The model under review builds one solid part; all positions refer to its coordinate system, in mm. Face numbers are marked on the shaded views. Round coordinates to 2 decimals unless told otherwise and drop trailing zeros. Order: outer loops, then holes, each group sorted by start corner. A loop starts at its lowest first (then second) coordinate and runs counter-clockwise, first axis right, second up.
1) Consider section D-D (y = 284). Give the boundary of the cut face in (x, z), then the cut area to 3 significant figures.
2) Consider section A-A (z = 12.7). Give the number of separate pieces and of enclosed holes in the cut face, then the cut area to 3 significant figures.
3) Mouldability with a two-part tool opening along Z and no side actions: class the marked faces 1 and 2 as pulls with the +Z half, pulls with the -Z half, needs draft (parallel to the pull), parting line crosses it, or undercut.
4) Consider section C-C (x = -18.25). Give the boundary of the cut face in (y, z).
5) Consider section B-B (y = 535.94). Give the boundary of the cut face in (x, z).
6) To check wall thickness, follow L1, parallel to Y at x = -24.45, z = 12.7; L2, parallel to X at y = 429.5, z = 19.25; L3, parallel to Z at x = -24.35, y = 322.58. State the ranges of each line that lie inside material, in increasing order.
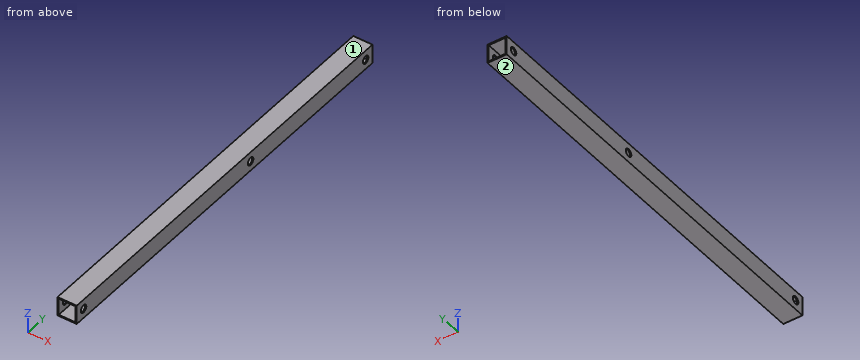
Autodesk Inventor part; units mm, degrees
ref_plane "YZ Plane" through (0, 0, 0) normal (1, 0, 0) x (0, 1, 0)
ref_plane "XZ Plane" through (0, 0, 0) normal (0, 1, 0) x (-1, 0, 0)
ref_plane "XY Plane" through (0, 0, 0) normal (0, 0, 1) x (1, 0, 0)
sketch "Sketch1" plane through (0, 0, 0) normal (0, 1, 0) x (-1, 0, 0)
  line L0 (0, 0) -> (25.4, 0)
  line L1 (25.4, 0) -> (25.4, 25.4)
  line L2 (25.4, 25.4) -> (0, 25.4)
  line L3 (0, 25.4) -> (0, 0)
  line L4 (23.8125, 23.8125) -> (1.5875, 23.8125)
  line L5 (1.5875, 23.8125) -> (1.5875, 1.5875)
  line L6 (1.5875, 1.5875) -> (23.8125, 1.5875)
  line L7 (23.8125, 1.5875) -> (23.8125, 23.8125)
  dimension "d0" = 25.4
  dimension "d1" = 25.4
  dimension "d2" = 1.5875
  dimension "d3" = 1.5875
  dimension "d4" = 1.5875
  dimension "d5" = 1.5875
extrude "Extrusion1" add sketch "Sketch1" along normal blind 548.64
sketch "Sketch2" plane through (0, 0, 25.4) normal (1, 0, 0) x (0, 0, -1)
  circle A0 centre (12.7, 12.7) radius 5.08
  line L0 (25.4, 0) -> (25.4, 548.64)
  line L1 (0, 0) -> (25.4, 0)
  dimension "d9" = 12.7
  dimension "d10" = 10.16
  dimension "d11" = 12.7
extrude "Extrusion2" cut sketch "Sketch2" against normal blind 25.4
sketch "Sketch3" plane through (0, 0, 25.4) normal (1, 0, 0) x (0, 0, -1)
  circle A0 centre (12.7, 535.94) radius 5.08
  line L0 (25.4, 0) -> (25.4, 548.64)
  line L1 (0, 548.64) -> (25.4, 548.64)
  dimension "d14" = 12.7
  dimension "d15" = 12.7
  dimension "d16" = 10.16
extrude "Extrusion3" cut sketch "Sketch3" against normal blind 25.4
sketch "Sketch4" plane through (0, 0, 25.4) normal (1, 0, 0) x (0, 0, -1)
  point P0 (25.4, 0)
sketch "Sketch5" plane through (0, 0, 25.4) normal (1, 0, 0) x (0, 0, -1)
  circle A0 centre (12.7, 322.58) radius 5.08
  line L0 (0, 0) -> (0, 548.64)
  circle A1 centre (12.7, 535.94) radius 5.08
  point P0 (25.4, 0)
  dimension "d19" = 10.16
  dimension "d20" = 12.7
  dimension "d21" = 213.36
extrude "Extrusion4" cut sketch "Sketch5" against normal blind 25.4 contours A0
properties part number "1x1 16th Inch Aluminum Tube - Custom for Lift Arms"
Answer below:
1. outline: (-25.4, 0) - (0, 0) - (0, 25.4) - (-25.4, 25.4) - close; hole (-23.81, 1.59) - (-1.59, 1.59) - (-1.59, 23.81) - (-23.81, 23.81) - close
1. area: 151 mm2
2. separate pieces: 8
2. enclosed holes: 0
2. area: 1,650 mm2
3. face 1: pulls with the +Z half
3. face 2: pulls with the -Z half
4. outline: (0, 0) - (548.64, 0) - (548.64, 1.59) - (0, 1.59) - close; (0, 23.81) - (548.64, 23.81) - (548.64, 25.4) - (0, 25.4) - close
5. outline: (-25.4, 0) - (0, 0) - (0, 7.62) - (-1.59, 7.62) - (-1.59, 1.59) - (-23.81, 1.59) - (-23.81, 7.62) - (-25.4, 7.62) - close; (-25.4, 17.78) - (-23.81, 17.78) - (-23.81, 23.81) - (-1.59, 23.81) - (-1.59, 17.78) - (0, 17.78) - (0, 25.4) - (-25.4, 25.4) - close
6. L1: y = 0 to 7.62, 17.78 to 317.5, 327.66 to 530.86, 541.02 to 548.64
6. L2: x = -25.4 to -23.81, -1.59 to 0
6. L3: z = 0 to 7.62, 17.78 to 25.4
